Design review of the part shown in the three views and the two pictorial views. Dimensions are in mm from the part's minimum x, y and z. Round coordinates to 2 decimals unless told otherwise and drop trailing zeros. Write each loop counter-clockwise with the first axis right and the second up, starting at its lowest first coordinate (ties: lowest second). Pieces come first, ordered by that corner, then holes. Notation, with made-up numbers: (44.25, 51.25) -> (89.25, 51.25) arc R21 cw to (89.25, 56.25) -> close; hole circle Ø7 at (28, -17.5). An arc over 180 degrees is marked (long way). Answer as a JSON object with one key per item and string values. Group by question number.
1) Insertion check: pin 1 Ø1 at (x, z) = (2.5, 2) entering from +Y; pin 2 Ø1 at (x, z) = (2, 1) entering from -Y; pin 3 Ø1 at (x, y) = (1.5, 127.5) entering from -Z (3 decimals). Each pin has a flat end and moves straight along its axis. Give the tip position at first contact, or say it passes through.
2) We need section B-B, the plane y = 72. Write out the cut boundary in (x, z) (1 decimal).
3) We need section A-A, the plane x = 1.9. Write out the cut boundary in (y, z) (1 decimal).
4) To check wall thickness, follow probe 1 along Y at (x, z) = (1, 1.75) (1 decimal); probe 2 along Z at (x, y) = (1.6, 103.5) (1 decimal). State the ranges of each line that lie inside material, in increasing order. Write a range as [from, to].
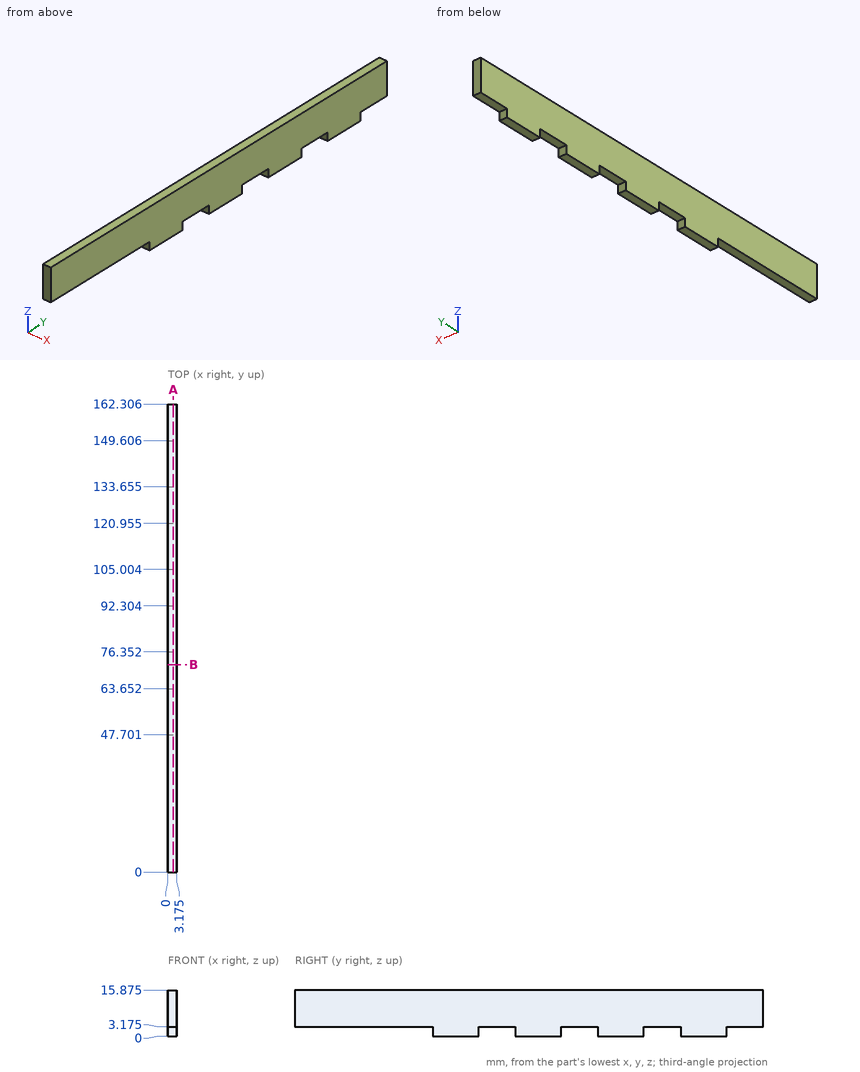
Here are the results:
{
 "1": {"pin 1": "stops at y = 149.61", "pin 2": "stops at y = 47.7", "pin 3": "stops at z = 3.175"},
 "2": {"outline": "(0, 3.2) -> (3.2, 3.2) -> (3.2, 15.9) -> (0, 15.9) -> close"},
 "3": {"outline": "(0, 3.2) -> (47.7, 3.2) -> (47.7, 0) -> (63.7, 0) -> (63.7, 3.2) -> (76.4, 3.2) -> (76.4, 0) -> (92.3, 0) -> (92.3, 3.2) -> (105, 3.2) -> (105, 0) -> (121, 0) -> (121, 3.2) -> (133.7, 3.2) -> (133.7, 0) -> (149.6, 0) -> (149.6, 3.2) -> (162.3, 3.2) -> (162.3, 15.9) -> (0, 15.9) -> close"},
 "4": {"probe 1": "y = [47.7, 63.7], [76.4, 92.3], [105, 121], [133.7, 149.6]", "probe 2": "z = [3.2, 15.9]"}
}
